Verification items for the finished model (mm, model axes). A direction names the side the tool comes from. Give positions to 0.01 mm unless a question says otherwise; leave off trailing zeros. Write each loop counter-clockwise with the first axis right and the second up, starting at its lowest first coordinate (ties: lowest second). Pieces come first, ordered by that corner, then holes.
from build123d import *

# Parameters (mm, degrees)
EXTRUDE_THIN1_DEPTH = 40
SKETCH2_R           = 6
CUT_EXTRUDE1_DEPTH  = 61
SKETCH3_R           = 6
CUT_EXTRUDE2_DEPTH  = 61


with BuildPart() as part:
    # Sketch1 → Extrude-Thin1 (new body, symmetric)
    with BuildSketch(Plane.XY):
        Polygon((60, 0), (0, 0), (0, 60), (5, 60), (5, 5), (60, 5), align=None)
    extrude(amount=EXTRUDE_THIN1_DEPTH, both=True)

    # Sketch2 → Cut-Extrude1 (cut, through all)
    with BuildSketch(Plane.XZ):
        with Locations((30, 0)):
            Circle(SKETCH2_R)
    extrude(amount=-CUT_EXTRUDE1_DEPTH, mode=Mode.SUBTRACT)

    # Sketch3 → Cut-Extrude2 (cut, through all)
    with BuildSketch(Plane(origin=(0, 0, 0), x_dir=(0, -1, 0), z_dir=(-1, 0, 0))):
        with Locations((-35, 0)):
            Circle(SKETCH3_R)
    extrude(amount=-CUT_EXTRUDE2_DEPTH, mode=Mode.SUBTRACT)


solid = part.part
Item 1: Sectioned sample at A-A on z = 0. Record the cut outline in (x, y), then the cut area to 3 significant figures.
Answer key:
outline: (0, 0) - (24, 0) - (24, 5) - (5, 5) - (5, 29) - (0, 29) - close; (0, 41) - (5, 41) - (5, 60) - (0, 60) - close; (36, 0) - (60, 0) - (60, 5) - (36, 5) - close
area: 455 mm2
Item 2: Set-up check for faces 4 (the face through (0, 23, 1)), 5 (the face through (5, 27, 1)): record each of +Z, -Z, +X, -X, +Y, -Y from which the full face is reachable in a straight line by a thin tool's end or side.
Answer key:
face 4: +Z, -Z, -X, +Y, -Y
face 5: +Z, -Z, +X, +Y
Item 3: Sectioned sample at D-D on z = -32. Record the cut outline in (x, y).
Answer key:
outline: (0, 0) - (60, 0) - (60, 5) - (5, 5) - (5, 60) - (0, 60) - close
Item 4: Sectioned sample at B-B on x = 30. Record the cut outline in (y, z), then the cut area to 3 significant figures.
Answer key:
outline: (0, -40) - (5, -40) - (5, -6) - (0, -6) - close; (0, 6) - (5, 6) - (5, 40) - (0, 40) - close
area: 340 mm2
Item 5: Release check for a two-part mould opening along Y. For faces 1 (the face through (37, 0, 1)), 2 (the face through (2, 41, 0)), 3 (the face through (17, 3, 40)) record: released by +Y, released by -Y, zero draft, split by the parting line, or undercut.
Answer key:
face 1: released by -Y
face 2: undercut
face 3: zero draft
Item 6: Depth check by flat-ended pin: pin 1 (12 mm diameter, centred on y = 23, z = -1, fed in from -X); pin 2 (1.5 mm diameter, centred on x = 42, z = -10.5, fed in from +Y); pin 3 (1 mm diameter, centred on y = 36, z = -29, fed in from +X); pin 4 (7 mm diameter, centred on y = 35, z = 0, fed in from -X). Enter the tip coordinate at first touch or a pass-through.
Answer key:
pin 1: stops at x = 0
pin 2: stops at y = 5
pin 3: stops at x = 5
pin 4: passes through
Item 7: Scan lines: line 1 along Z through (x, y) = (1.5, 35); line 2 along Y through (x, z) = (18.5, 5.5). Record each from-to range of solid material in increasing order.
Answer key:
line 1: z = -40 to -6, 6 to 40
line 2: y = 0 to 5
